Work out the finished part from the listing and answer in its coordinate system (mm). A direction names the side the tool comes from. Round coordinates to 2 decimals unless told otherwise and drop trailing zeros. Write each loop counter-clockwise with the first axis right and the second up, starting at its lowest first coordinate (ties: lowest second). Pieces come first, ordered by that corner, then holes. Notation, with made-up numbers: M 37,57.25 L 68,57.25 A22 cw 68,78.25 Z; hole C 34.5,-13 d8. An arc over 180 degrees is marked long. One line per item, written item: value. Start each with the question number.
Q1. A tool of negligible diameter and unlimited length cuts with its end or side. For faces 4 (the flat face through (-1, 11, -13.009)), 5 (the flat face through (7, 2, -61)), 6 (the cylindrical face through (-0.681, 4.986, -12.863)), 7 (the flat face through (3, 2, 7.579)), from which of +Z, -Z, +X, -X, +Y, -Y can it reach the whole face along a straight path? Write none if from no direction.
Q2. Find section B-B (x = 12.75). Write down the section's boundary in (y, z), and give its area (3 significant figures).
Q3. Given pin 1 Ø1 at (y, z) = (13.5, -49) entering from -X; pin 2 Ø0.6 at (x, y) = (-3.5, 7.5) entering from -Z; pin 3 Ø1.1 at (x, z) = (1.5, -55.5) entering from +Y, each flat-ended and moving along its own axis, determine where each tip first touches the part or whether it passes through.
Q4. The mould has two halves that part along Y. Classify faces 1 (the flat face through (11, 12, -41)), 2 (the flat face through (0, 7, -41)), 3 (the cylindrical face through (13.54, 11.53, -49.85)): released by +Y, released by -Y, zero draft, split by the parting line, or undercut.
Q5. Consider probe 1 along Z at (x, y) = (0.75, 5.75); probe 2 along Y at (x, z) = (14.75, -10.5); probe 3 along X at (y, z) = (11.5, 8.5). Determine where each line is inside the solid, lowest interval first.
Q6. Find section A-A (z = 10.5). Write down the section's boundary in (x, y).
Q7. Find section C-C (y = 11). Count the separate pieces of the cut face and the enclosed holes in it, and give its area (3 significant figures).
from build123d import *

# Parameters (mm, degrees)
BOSS_EXTRUDE1_DEPTH = 11
SKETCH3_W           = 22
SKETCH3_H           = 3
BOSS_EXTRUDE2_DEPTH = 14
BOSS_EXTRUDE3_DEPTH = 5
SKETCH5_R           = 1.75
CUT_EXTRUDE1_DEPTH  = 36.096650541
SKETCH6_W           = 9
SKETCH6_H           = 9
BOSS_EXTRUDE4_DEPTH = 5
SKETCH10_R          = 2.25
CUT_EXTRUDE2_DEPTH  = 34.584744739
SKETCH8_W           = 27
SKETCH8_H           = 15.7
BOSS_EXTRUDE5_DEPTH = 4.5
FILLET1_R           = 0.75
CUT_EXTRUDE3_DEPTH  = 4
SKETCH12_R          = 1.5
CUT_EXTRUDE4_DEPTH  = 2


with BuildPart() as part:
    # Sketch1 → Boss-Extrude1 (new, symmetric)
    with BuildSketch(Plane(origin=(0, 0, 0), x_dir=(0, 0, -1), z_dir=(1, 0, 0))):
        Polygon((-13.0089, 0), (13.0089, 0), (13.0089, 8.5), (5.7589, 8.5), (5.7589, 7), (-5.7589, 7), (-5.7589, 8.5), (-13.0089, 8.5), align=None)
    extrude(amount=BOSS_EXTRUDE1_DEPTH, both=True)

    # Sketch3 → Boss-Extrude2 (add)
    with BuildSketch(Plane.XZ):
        with Locations((0, -14.5089)):
            Rectangle(SKETCH3_W, SKETCH3_H)
        with Locations((0, 14.5089)):
            Rectangle(SKETCH3_W, SKETCH3_H)
    extrude(amount=-BOSS_EXTRUDE2_DEPTH)

    # Sketch4 → Boss-Extrude3 (add)
    with BuildSketch(Plane(origin=(11, 0, 0), x_dir=(0, 0, -1), z_dir=(1, 0, 0))):
        Polygon((-8.8, 15.7), (-16.0089, 15.7), (-16.0089, 0), (16.0089, 0), (16.0089, 15.7), align=None)
    extrude(amount=BOSS_EXTRUDE3_DEPTH)

    # Sketch5 → Cut-Extrude1 (cut, through all)
    with BuildSketch(Plane(origin=(16, 0, 0), x_dir=(0, 0, -1), z_dir=(1, 0, 0))):
        with Locations((-10.5, 11)):
            Circle(SKETCH5_R)
        with Locations((10.5, 11)):
            Circle(SKETCH5_R)
    extrude(amount=-CUT_EXTRUDE1_DEPTH, mode=Mode.SUBTRACT)

    # Sketch6 → Boss-Extrude4 (add)
    with BuildSketch(Plane.XZ):
        with Locations((11.5, 20.5089)):
            Rectangle(SKETCH6_W, SKETCH6_H)
    extrude(amount=-BOSS_EXTRUDE4_DEPTH)

    # Sketch10 → Cut-Extrude2 (cut, through all)
    with BuildSketch(Plane.XZ):
        with Locations(Location((11.5, 20.5089, 0), (0, 0, 270))):
            Circle(SKETCH10_R)
    extrude(amount=-CUT_EXTRUDE2_DEPTH, mode=Mode.SUBTRACT)

    # Sketch8 → Boss-Extrude5 (add)
    with BuildSketch(Plane(origin=(0, 0, -16.0089), x_dir=(-1, 0, 0), z_dir=(0, 0, -1))):
        with Locations((-2.5, 7.85)):
            Rectangle(SKETCH8_W, SKETCH8_H)
    extrude(amount=BOSS_EXTRUDE5_DEPTH)

    # Fillet1
    fillet1_edges = [part.edges().sort_by_distance(p)[0] for p in [
        (0, 8.5, 5.7589),
        (0, 8.5, -5.7589),
        (0, 14, -13.0089),
        (11, 14, -14.5089),
        (11, 11.25, -13.0089),
        (11, 14, 14.5089),
        (11, 11.25, 13.0089),
        (0, 14, 13.0089),
        (11, 15.7, 0),
        (16, 15.7, -2.25),
        (11.5, 5, 25.0089),
    ]]
    fillet(fillet1_edges, radius=FILLET1_R)

    # Mirror6: part across plane


with BuildPart() as part_1:
    add(part.part)
    add(part.part.mirror(Plane(origin=(0, 0, -20.5089), x_dir=(1, 0, 0), z_dir=(0, 0, -1))))

    # Sketch11 → Cut-Extrude3 (cut)
    with BuildSketch(Plane.XZ):
        Polygon((0.65, 7.5789), (16, 7.5789), (16, -31.9211), (-11, -31.9211), (-11, 7.5789), align=None)
    extrude(amount=-CUT_EXTRUDE3_DEPTH, mode=Mode.SUBTRACT)

    # Sketch12 → Cut-Extrude4 (cut)
    with BuildSketch(Plane.XZ.offset(-4)):
        with Locations(Location((0.65, -12.1711, 0), (0, 0, 270))):
            Circle(SKETCH12_R)
    extrude(amount=-CUT_EXTRUDE4_DEPTH, mode=Mode.SUBTRACT)


solid = part_1.part
The answers:
1. face 4: -X, +Y
1. face 5: -Z, -X, +Y, -Y
1. face 6: -Y
1. face 7: +X, -X, -Y
2. outline: M 0,-66.03 L 4.25,-66.03 A0.75 ccw 5,-65.28 L 5,-63.4 L 0,-63.4 Z; M 0,-59.66 L 5,-59.66 L 5,-57.03 L 15.7,-57.03 L 15.7,16.01 L 5,16.01 L 5,18.64 L 0,18.64 L 0,7.58 L 4,7.58 L 4,-31.92 L 0,-31.92 Z; M 0,22.38 L 5,22.38 L 5,24.26 A0.75 ccw 4.25,25.01 L 0,25.01 Z; hole C 11,-51.52 d3.5; hole C 11,-30.52 d3.5; hole C 11,-10.5 d3.5; hole C 11,10.5 d3.5
2. area: 1,000 mm2
3. pin 1: x = 11
3. pin 2: z = -57.03
3. pin 3: y = 14
4. face 1: zero draft
4. face 2: released by +Y
4. face 3: undercut
5. probe 1: -57.03 to -13.67, -10.67 to 16.01
5. probe 2: 4 to 9.25, 12.75 to 15.7
5. probe 3: 11 to 16
6. outline: M -11,0 L 16,0 L 16,9.25 L 11,9.25 L 11,8.5 L -11,8.5 Z; M 11,12.75 L 16,12.75 L 16,14.95 A0.75 ccw 15.25,15.7 L 11.75,15.7 A0.75 ccw 11,14.95 Z
7. separate pieces: 5
7. enclosed holes: 0
7. area: 758 mm2
